For this review, take the finished solid that the model builds, in its own axes (mm). Face numbers are marked on the shaded views. A direction names the side the tool comes from. Coordinates: 2 decimals unless noted, no trailing zeros. Write each loop counter-clockwise with the first axis right and the second up, starting at its lowest first coordinate (ties: lowest second). Pieces come first, ordered by that corner, then holes. Notation, with made-up numbers: M -7.5,32 L 41.5,32 A23 ccw 41.5,42 Z; hole C 86,-13.5 d11. An arc over 180 degrees is marked long. Return JSON: item names as keys, results as strings.
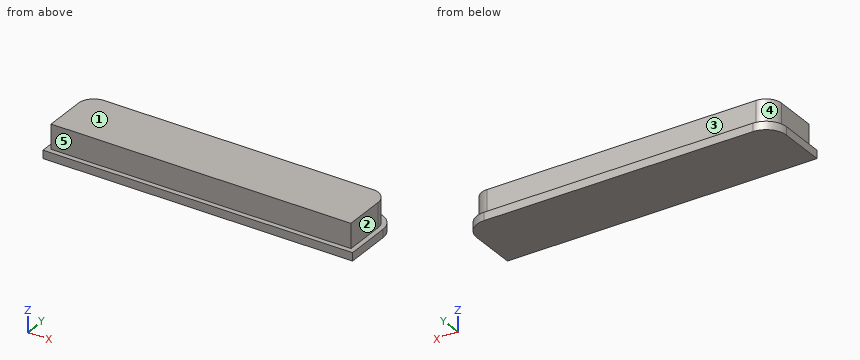
```python
from build123d import *

# Parameters (mm, degrees)
BOSS_EXTRUDE1_DEPTH = 1
BOSS_EXTRUDE2_DEPTH = 3


with BuildPart() as part:
    # Sketch1 → Boss-Extrude1 (new body)
    with BuildSketch(Plane.XY):
        with BuildLine():
            Line((0, 0), (0, 5.7))
            ThreePointArc((0, 5.7), (0.732233047, 7.467766953), (2.5, 8.2))
            Line((2.5, 8.2), (35.5, 8.2))
            ThreePointArc((35.5, 8.2), (37.267766953, 7.467766953), (38, 5.7))
            Line((38, 5.7), (38, 0))
            Line((38, 0), (0, 0))
        make_face()
    extrude(amount=BOSS_EXTRUDE1_DEPTH)

    # Sketch2 → Boss-Extrude2 (add)
    with BuildSketch(Plane.XY.offset(1)):
        with BuildLine():
            Line((0.6, 0.6), (0.6, 5.7))
            ThreePointArc((0.6, 5.7), (1.156497116, 7.043502884), (2.5, 7.6))
            Line((2.5, 7.6), (35.5, 7.6))
            ThreePointArc((35.5, 7.6), (36.843502884, 7.043502884), (37.4, 5.7))
            Line((37.4, 5.7), (37.4, 0.6))
            Line((37.4, 0.6), (0.6, 0.6))
        make_face()
    extrude(amount=BOSS_EXTRUDE2_DEPTH)


solid = part.part
```
1. For the marked faces 1, 2, 3, 4 and 5, list the 3-axis set-ups (+Z, -Z, +X, -X, +Y, -Y) from which the entire face can be reached by the end or side of a thin tool; tool diameter is ignored.
Checks:
{"face 1": "+Z, +X, -X, +Y, -Y", "face 2": "+Z, +X, +Y, -Y", "face 3": "+Z, +X, -X, +Y", "face 4": "+Z, -X, +Y", "face 5": "+Z, +X, -X, -Y"}
2. We need section C-C (z = 1.95). State the section outline as (x, y) points.
Checks:
{"outline": "M 0.6,0.6 L 37.4,0.6 L 37.4,5.7 A1.9 ccw 35.5,7.6 L 2.5,7.6 A1.9 ccw 0.6,5.7 Z"}
3. We need section B-B (y = 4.5). State the section outline as (x, z) points, plus the area to 3 significant figures.
Checks:
{"outline": "M 0,0 L 38,0 L 38,1 L 37.4,1 L 37.4,4 L 0.6,4 L 0.6,1 L 0,1 Z", "area": "148 mm2"}
4. Clearance check with flat-ended pins moving along their axes: pin 1 Ø1 at (x, z) = (19.5, 2.5) entering from -Y; pin 2 Ø1.5 at (x, z) = (27, 2) entering from +Y; pin 3 Ø1.5 at (y, z) = (3.5, 3) entering from +X. State where each tip first meets the part, or that it passes through.
Checks:
{"pin 1": "y = 0.6", "pin 2": "y = 7.6", "pin 3": "x = 37.4"}
5. Wall thickness on L1, parallel to X at y = 4.5, z = 2; L2, parallel to Y at x = 29.5, z = 3.4; L3, parallel to Z at x = 25, y = 7.75: over which ranges is each line inside the solid? List them lowest first. Write a range as from..to.
Checks:
{"L1": "0.6..37.4", "L2": "0.6..7.6", "L3": "0..1"}
6. We need section A-A (x = 5). State the section outline as (y, z) points, plus the area to 3 significant figures.
Checks:
{"outline": "M 0,0 L 8.2,0 L 8.2,1 L 7.6,1 L 7.6,4 L 0.6,4 L 0.6,1 L 0,1 Z", "area": "29.2 mm2"}
